from build123d import *

# Parameters (mm, degrees)
SKETCH_W       = 58
SKETCH_H       = 82.5
PAD_DEPTH      = 22
PAD_DEPTH_BACK = 22
SKETCH001_R    = 12.5
PAD001_DEPTH   = 5
SKETCH002_R    = 5
PAD002_DEPTH   = 20
SKETCH003_R    = 4
PAD003_DEPTH   = 2.5
FILLET_R       = 2
SKETCH004_R    = 22
PAD004_DEPTH   = 66.53
SKETCH005_W    = 68
SKETCH005_H    = 85
PAD005_DEPTH   = 5
SKETCH006_W    = 5
SKETCH006_H    = 85
PAD006_DEPTH   = 50


with BuildPart() as part:
    # Sketch → Pad (new body, two sides)
    with BuildSketch(Plane.XY) as pad_sk:
        with Locations((29, -41.25)):
            Rectangle(SKETCH_W, SKETCH_H)
    extrude(amount=PAD_DEPTH)
    extrude(pad_sk.sketch, amount=-PAD_DEPTH_BACK)

    # Sketch001 (on Face6 of Pad) → Pad001 (join)
    with BuildSketch(Plane.XY.offset(22)):
        with Locations((29, -23.5)):
            Circle(SKETCH001_R)
    pad001 = extrude(amount=PAD001_DEPTH)

    # Mirrored: Pad001 across XY
    add(pad001.mirror(Plane.XY))

    # Sketch002 (on Face10 of Mirrored) → Pad002 (join)
    with BuildSketch(Plane.XY.offset(27)):
        with Locations((29, -23.5)):
            Circle(SKETCH002_R)
    pad002 = extrude(amount=PAD002_DEPTH)

    # Mirrored001: Pad002 across XY
    add(pad002.mirror(Plane.XY))

    # Sketch003 (on Face5 of Mirrored001) → Pad003 (join)
    with BuildSketch(Plane.XY.offset(22)):
        with Locations((10, -12.57)):
            Circle(SKETCH003_R)
        with Locations((48, -12.57)):
            Circle(SKETCH003_R)
        with Locations((10, -68.57)):
            Circle(SKETCH003_R)
        with Locations((48, -54.57)):
            Circle(SKETCH003_R)
    pad003 = extrude(amount=PAD003_DEPTH)

    # Mirrored002: Pad003 across XY
    add(pad003.mirror(Plane.XY))

    # Fillet
    fillet_edges = [part.edges().sort_by_distance(p)[0] for p in [
        (58, 0, 0),
        (0, 0, 0),
        (58, -82.5, 0),
        (0, -82.5, 0),
    ]]
    fillet(fillet_edges, radius=FILLET_R)

    # Sketch004 (on Face10 of Fillet) → Pad004 (join)
    with BuildSketch(Plane.XZ.offset(82.5)):
        with Locations((29, 0)):
            Circle(SKETCH004_R)
    extrude(amount=PAD004_DEPTH)

    # Sketch005 (on Face32 of Pad004) → Pad005 (join)
    with BuildSketch(Plane.XY.offset(24.5)):
        with Locations((34, -42.5)):
            Rectangle(SKETCH005_W, SKETCH005_H)
        with BuildLine():
            ThreePointArc((43, -23.5), (29, -9.5), (15, -23.5))
            Line((15, -23.5), (15, -48.5))
            ThreePointArc((15, -48.5), (29, -62.5), (43, -48.5))
            Line((43, -48.5), (43, -23.5))
        make_face(mode=Mode.SUBTRACT)
    extrude(amount=PAD005_DEPTH)

    # Sketch006 (on Face4 of Pad005) → Pad006 (join)
    with BuildSketch(Plane(origin=(0, 0, 24.5), x_dir=(1, 0, 0), z_dir=(0, 0, -1))):
        with Locations((65.5, 42.5)):
            Rectangle(SKETCH006_W, SKETCH006_H)
    extrude(amount=PAD006_DEPTH)


solid = part.part
The model under review builds one solid part; all positions refer to its coordinate system, in mm. A direction names the side the tool comes from. Give positions to 0.01 mm unless a question says otherwise; leave off trailing zeros. Order: outer loops, then holes, each group sorted by start corner. A loop starts at its lowest first (then second) coordinate and runs counter-clockwise, first axis right, second up. Notation, with made-up numbers: M 84.25,83.25 L 131.25,83.25 A14 ccw 131.25,101.25 Z; hole C -29.75,-21 d10. An arc over 180 degrees is marked long. Answer in a Markdown table with one row per item. Add a question column.
1. Add section B-B on x = 46.5. State the section outline as (y, z) points, plus the area to 3 significant figures.
2. For pin 1 Ø6.5 at (x, y) = (49.5, -55) entering from -Z; pin 2 Ø17.5 at (x, y) = (16, -45.5) entering from -Z; pin 3 Ø12 at (x, y) = (59.5, -28.5) entering from -Z, all flat-tipped, find the tip position at first contact; note any pin that passes through.
3. Machinability: for faces 1 (the flat face through (29, -29, -27)), 2 (the flat face through (29, -29, 27)), 3 (the flat face through (46, -85, 25)), which of the approach directions +Z, -Z, +X, -X, +Y, -Y give a long, thin tool a straight path to every point of the face, cutting with its end or side? Answer none if there is none.
4. Add section A-A on y = -44. State the section outline as (x, z) points, plus the area to 3 significant figures.
5. Mouldability with a two-part tool opening along Z and no side actions: class faces 4 (the cylindrical face through (25, -26.5, 36.9)), 5 (the flat face through (10, -69, -24.5)), 6 (the cylindrical face through (7.05, -9.87, 23.23)) as released by +Z, released by -Z, zero draft, split by the parting line, or undercut.
6. Add section D-D on z = -29. State the section outline as (x, y) points, plus the area to 3 significant figures.
7. Add section C-C on x = 19.5. State the section outline as (y, z) points.
8. To check wall thickness, follow line 1 along Z through (x, y) = (46, -67.5); line 2 along X through (y, z) = (-50, 7); line 3 along Z through (x, y) = (29, -118.5). State the ranges of each line that lie inside material, in increasing order.
The answers:
| question | item | result |
|---|---|---|
| 1 | outline | M -149.03,-13.33 L -82.5,-13.33 L -82.5,-22 L -58.28,-22 L -58.28,-24.5 L -50.86,-24.5 L -50.86,-22 L -16.28,-22 L -16.28,-24.5 L -8.86,-24.5 L -8.86,-22 L 0,-22 L 0,22 L -8.86,22 L -8.86,24.5 L 0,24.5 L 0,29.5 L -85,29.5 L -85,24.5 L -58.28,24.5 L -58.28,22 L -82.5,22 L -82.5,13.33 L -149.03,13.33 Z; hole M -50.86,22 L -16.28,22 L -16.28,24.5 L -50.86,24.5 Z |
| 1 | area | 5,900 mm2 |
| 2 | pin 1 | z = -24.5 |
| 2 | pin 2 | z = -22 |
| 2 | pin 3 | z = -25.5 |
| 3 | face 1 | -Z |
| 3 | face 2 | +Z |
| 3 | face 3 | +Z, +X, -Y |
| 4 | outline | M 0,-22 L 58,-22 L 58,22 L 0,22 Z; M 0,24.5 L 15,24.5 L 15,29.5 L 0,29.5 Z; M 43,24.5 L 63,24.5 L 63,-25.5 L 68,-25.5 L 68,29.5 L 43,29.5 Z |
| 4 | area | 3,000 mm2 |
| 5 | face 4 | zero draft |
| 5 | face 5 | released by -Z |
| 5 | face 6 | undercut |
| 6 | outline | C 29,-23.5 d10 |
| 6 | area | 78.5 mm2 |
| 7 | outline | M -149.03,-19.84 L -82.5,-19.84 L -82.5,-22 L -31.62,-22 L -31.62,-27 L -15.38,-27 L -15.38,-22 L 0,-22 L 0,22 L -15.38,22 L -15.38,27 L -31.62,27 L -31.62,22 L -82.5,22 L -82.5,19.84 L -149.03,19.84 Z; M -85,24.5 L -58.78,24.5 L -58.78,29.5 L -85,29.5 Z; M -13.22,24.5 L 0,24.5 L 0,29.5 L -13.22,29.5 Z |
| 8 | line 1 | -22 to 22, 24.5 to 29.5 |
| 8 | line 2 | 0 to 58, 63 to 68 |
| 8 | line 3 | -22 to 22 |
